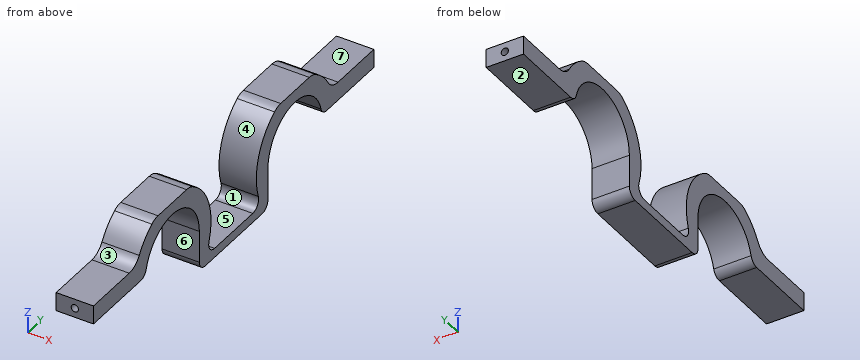
Autodesk Inventor part; units mm, degrees
ref_plane "YZ Plane" through (0, 0, 0) normal (1, 0, 0) x (0, 1, 0)
ref_plane "XZ Plane" through (0, 0, 0) normal (0, 1, 0) x (-1, 0, 0)
ref_plane "XY Plane" through (0, 0, 0) normal (0, 0, 1) x (1, 0, 0)
sketch "Sketch1" plane through (0, 0, 0) normal (1, 0, 0) x (0, 1, 0)
  line L0 (-11.75, 0.3) -> (11.75, 0.3)
  arc A0 (30.2011, 10.1) -> (11.75, 9.15) centre (21, 9.15) ccw
  arc A1 (-11.75, 9.15) -> (-30.2011, 10.1) centre (-21, 9.15) ccw
  line L1 (-30.2011, 10.1) -> (-48, 10.1)
  line L2 (-48, 10.1) -> (-48, 14.1)
  line L3 (-48, 14.1) -> (-33.2906, 14.1)
  arc A2 (-8.4379, 4.9361) -> (-33.2906, 14.1) centre (-21, 9.15) ccw
  arc A3 (33.2906, 14.1) -> (8.4379, 4.9361) centre (21, 9.15) ccw
  line L4 (30.2011, 10.1) -> (48, 10.1)
  line L5 (48, 10.1) -> (48, 14.1)
  line L6 (48, 14.1) -> (33.2906, 14.1)
  line L7 (6.5418, 2.3) -> (-6.5418, 2.3)
  line L8 (-26.9279, 21) -> (-15.0721, 21)
  line L9 (15.0721, 21) -> (26.9279, 21)
  line L10 (11.75, 9.15) -> (11.75, 0.3)
  line L11 (-11.75, 9.15) -> (-11.75, 0.3)
  arc A4 (-8.4379, 4.9361) -> (-6.5418, 2.3) centre (-6.5418, 4.3) ccw
  arc A5 (6.5418, 2.3) -> (8.4379, 4.9361) centre (6.5418, 4.3) ccw
  point P0 (0, 0)
  point P1 (0, 0.3)
  point P2 (0, 2.3)
  dimension "d1" = 9.25
  dimension "d3" = 42
  dimension "d4" = 96
  dimension "d5" = 4
  dimension "d8" = 4
  dimension "d11" = 0.3
  dimension "d13" = 10.1
  dimension "d14" = 9.15
  dimension "d15" = 21
  dimension "d26" = 2
  dimension "d30" = 2
  dimension "d31" = 13.0836
extrude "Extrusion1" add sketch "Sketch1" along normal mid plane 8 contours L11 A1 L1 L2 L3 A2 L8 A4 L7 A5 A3 L9 L6 L5 L4 A0 L10 L0
sketch "Sketch2" plane through (-4, 48, 14.1) normal (0, 1, 0) x (1, 0, 0)
  line L0 (0, 0) -> (8, 0)
  line L1 (8, 4) -> (8, 0)
  line L2 (0, 4) -> (8, 4)
  line L3 (0, 0) -> (0, 4)
  line L4 (0, 4) -> (8, 4)
  line L5 (0, 0) -> (0, 4)
  point P0 (4, 14.1)
  point P1 (4, 2)
  point P2 (4, 4)
  point P3 (0, 2)
hole "Hole1" at (0, 48, 12.1) direction (0, -1, 0) diameter 1.567 depth 6.3 tip angle 118
mirror "Mirror1" about plane through (0, 0, 0) normal (0, 1, 0) of "Hole1"
fillet "Fillet3" radius 4 6 edges at (0, -26.9279, 21) (0, -15.0721, 21) (0, 15.0721, 21) (0, 26.9279, 21) (0, 33.2906, 14.1) (0, -33.2906, 14.1)
fillet "Fillet3" radius 2 4 edges at (0, -30.2011, 10.1) (0, 30.2011, 10.1) (0, -11.75, 0.3) (0, 11.75, 0.3)
properties part number "EPS_RegulatorHeatsinkBatteryAdapter" material "Copper"
Verification items for the finished model (mm, model axes). Face numbers are marked on the shaded views. A direction names the side the tool comes from. Coordinates: 2 decimals unless noted, no trailing zeros. Order: outer loops, then holes, each group sorted by start corner. A loop starts at its lowest first (then second) coordinate and runs counter-clockwise, first axis right, second up. Notation, with made-up numbers: (-33.5, -1) - (-24.5, -1) arc R20 ccw to (-24.5, 37) - close; hole circle Ø11 at (-20, 88.5). An arc over 180 degrees is marked (long way). Return JSON: item names as keys, results as strings.
(1) Thickness scan on line 1 along X through (y, z) = (43.75, 12.1); line 2 along Z through (x, y) = (0, -45.5); line 3 along Y through (x, z) = (-3.5, 11.25). Record the ranges inside material, lowest first.
Filled sheet:
{"line 1": "x = -4 to -0.78, 0.78 to 4", "line 2": "z = 10.1 to 11.32, 12.88 to 14.1", "line 3": "y = -48 to -30.05, -11.99 to -7.92, 7.92 to 11.99, 30.05 to 48"}
(2) Access from +Z, -Z, +X, -X, +Y, -Y to the whole of each face (thin tool, end or side, straight path). Record for the marked faces 4, 5, 6 and 7.
Filled sheet:
{"face 4": "+X, -X", "face 5": "+Z, +X, -X", "face 6": "-Z, +X, -X, -Y", "face 7": "+Z, +X, -X, +Y"}
(3) Section check C-C, the plane y = 2. Record the cut outline in (x, z), and give its area (3 significant figures).
Filled sheet:
{"outline": "(-4, 0.3) - (4, 0.3) - (4, 2.3) - (-4, 2.3) - close", "area": "16.0 mm^2"}
(4) Mould release check, pull along Z, two halves, no side actions. Record for the marked faces 1, 2 and 3: pulls with the +Z half, pulls with the -Z half, needs draft (parallel to the pull), parting line crosses it, or undercut.
Filled sheet:
{"face 1": "undercut", "face 2": "pulls with the -Z half", "face 3": "pulls with the +Z half"}
(5) Section check A-A, the plane z = 7.25. Record the cut outline in (x, y).
Filled sheet:
{"outline": "(-4, -11.75) - (4, -11.75) - (4, -7.89) - (-4, -7.89) - close; (-4, 7.89) - (4, 7.89) - (4, 11.75) - (-4, 11.75) - close"}
(6) Section check D-D, the plane z = 19.5. Record the cut outline in (x, y), and give its area (3 significant figures).
Filled sheet:
{"outline": "(-4, -29.27) - (4, -29.27) - (4, -12.73) - (-4, -12.73) - close; (-4, 12.73) - (4, 12.73) - (4, 29.27) - (-4, 29.27) - close", "area": "265 mm^2"}
(7) Go/stop test with flat-tipped pins: pin 1 (1.4 mm diameter, centred on x = 0, z = 12.1, fed in from -Y); pin 2 (0.9 mm diameter, centred on x = 0, z = 12.1, fed in from -Y); pin 3 (4 mm diameter, centred on x = 1, y = 40, fed in from -Z). Record where each tip stops, or that it passes through.
Filled sheet:
{"pin 1": "stops at y = -41.65", "pin 2": "stops at y = -41.5", "pin 3": "stops at z = 10.1"}
